from build123d import *

# Parameters (mm, degrees)
REVOLVE1_ANGLE = 270


with BuildPart() as part:
    # Sketch1 → Revolve1 (revolve)
    with BuildSketch(Plane.XY):
        with BuildLine():
            Line((0, 40.288428911), (70, 40.288428911))
            ThreePointArc((70, 40.288428911), (77.071067812, 37.359496723), (80, 30.288428911))
            Line((80, 30.288428911), (80, -204.742322884))
            Line((80, -204.742322884), (100, -204.742322884))
            Line((100, -204.742322884), (100, 45.257677116))
            ThreePointArc((100, 45.257677116), (97.071067812, 52.328744927), (90, 55.257677116))
            Line((90, 55.257677116), (0, 55.257677116))
            Line((0, 55.257677116), (0, 40.288428911))
        make_face()
    revolve(axis=Axis((0, 40.288428911, 0), (0, -1, 0)), revolution_arc=REVOLVE1_ANGLE)


solid = part.part
Model file for the job. Use its own axes, mm. A direction names the side the tool comes from. Round coordinates to 2 decimals unless told otherwise and drop trailing zeros. Loops run counter-clockwise (first coordinate to the right, second up) from the corner with the lowest first, then second, coordinate; pieces in that order, holes last. Notation, with made-up numbers: (-4.5, -21) - (28.5, -21) arc R19 ccw to (28.5, -2) - close; hole circle Ø2 at (34, 16). An arc over 180 degrees is marked (long way). Write each question's results on one line, items separated by ' | '.
(1) Saw through at A-A, the plane y = -9. List the corners of the cut face in (x, z).
Answer below:
outline: (0, -100) - (0, -80) arc R80 cw (long way) to (80, 0) - (100, 0) arc R100 ccw (long way) to start
(2) Wall check: L1, parallel to X at y = 2, z = 10.5; L2, parallel to X at y = 13, z = 53.5; L3, parallel to Y at x = 8, z = 14.5. Give the ranges that are in metal, low to high.
Answer below:
L1: x = -99.45 to -79.31, 79.31 to 99.45 | L2: x = -84.49 to -59.48, 59.48 to 84.49 | L3: y = 40.29 to 55.26
(3) 3-axis set-ups, long thin cutter, end or side, ignore diameter. For faces 1 (the cylindrical face through (-54.672, -88.872, 58.403)), 2 (the flat face through (-1, 55.258, 1)), 3 (the flat face through (83, -45, 0)): which of +Z, -Z, +X, -X, +Y, -Y reach the whole face in a straight line?
Answer below:
face 1: -Y | face 2: +Z, -Z, +X, -X, +Y | face 3: -Z, +X, +Y, -Y
(4) Pin check, flat tips, straight feed: pin 1 (3 mm diameter, centred on x = -58, z = -30, fed in from -Y); pin 2 (6 mm diameter, centred on x = 40, y = -151, fed in from +Z); pin 3 (12 mm diameter, centred on x = 4, y = -10.5, fed in from -Z); pin 4 (3 mm diameter, centred on y = -89, z = 59, fed in from +X). Stop position of each tip, or through.
Answer below:
pin 1: stops at y = 40.29 | pin 2: stops at z = 92.9 | pin 3: stops at z = -100 | pin 4: stops at x = 81.82
